Autodesk Inventor part; units mm, degrees
ref_plane "YZ Plane" through (0, 0, 0) normal (1, 0, 0) x (0, 1, 0)
ref_plane "XZ Plane" through (0, 0, 0) normal (0, 1, 0) x (-1, 0, 0)
ref_plane "XY Plane" through (0, 0, 0) normal (0, 0, 1) x (1, 0, 0)
sketch "Boceto1" plane through (0, 0, 0) normal (0, 0, 1) x (1, 0, 0)
  line L0 (0, 0) -> (130, 0)
  line L1 (130, 0) -> (130, -56.08)
  line L2 (130, -56.08) -> (0, -56.08)
  line L3 (0, -56.08) -> (0, 0)
  dimension "d0" = 130
  dimension "d1" = 56.08
extrude "Extrusión1" add sketch "Boceto1" along normal blind 5
sketch "Boceto2" plane through (0, 0, 5) normal (0, 0, 1) x (1, 0, 0)
  line L0 (130, 0) -> (130, -56.08)
  line L1 (0, -56.08) -> (0, 0)
  line L2 (130, -56.08) -> (0, -56.08)
  line L3 (16.75, -57.2435) -> (13.25, -57.2435)
  line L4 (13.25, -44.08) -> (16.75, -44.08)
  line L5 (116.75, -57.2435) -> (113.25, -57.2435)
  line L6 (113.25, -44.08) -> (116.75, -44.08)
  line L7 (12, -46.6661) -> (12, -49.2661)
  line L8 (18, -49.2661) -> (18, -46.6661)
  line L9 (112, -46.6661) -> (112, -49.2661)
  line L10 (118, -49.2661) -> (118, -46.6661)
  line L11 (12, -49.2661) -> (13.25, -49.2661)
  line L12 (16.75, -49.2661) -> (18, -49.2661)
  line L13 (16.75, -44.08) -> (16.75, -46.6661)
  line L14 (16.75, -49.2661) -> (16.75, -57.2435)
  line L15 (18, -46.6661) -> (16.75, -46.6661)
  line L16 (13.25, -46.6661) -> (12, -46.6661)
  line L17 (13.25, -57.2435) -> (13.25, -49.2661)
  line L18 (13.25, -46.6661) -> (13.25, -44.08)
  line L19 (112, -49.2661) -> (113.25, -49.2661)
  line L20 (116.75, -49.2661) -> (118, -49.2661)
  line L21 (116.75, -44.08) -> (116.75, -46.6661)
  line L22 (116.75, -49.2661) -> (116.75, -57.2435)
  line L23 (118, -46.6661) -> (116.75, -46.6661)
  line L24 (113.25, -46.6661) -> (112, -46.6661)
  line L25 (113.25, -57.2435) -> (113.25, -49.2661)
  line L26 (113.25, -46.6661) -> (113.25, -44.08)
  dimension "d7" = 6
  dimension "d8" = 12
  dimension "d14" = 13.25
  dimension "d15" = 1.25
  dimension "d16" = 1.25
  dimension "d17" = 13.25
  dimension "d18" = 3.5
extrude "Extrusión2" cut sketch "Boceto2" against normal blind 5
sketch "Boceto3" plane through (0, 0, 5) normal (0, 0, 1) x (1, 0, 0)
  line L0 (0, -56.08) -> (0, 0)
  line L1 (63.25, -6.5636) -> (63.25, 0.2503)
  line L2 (66.75, 0.2503) -> (66.75, -6.5636)
  line L3 (66.75, -6.5636) -> (68, -6.5636)
  line L4 (68, -6.5636) -> (68, -9.1636)
  line L5 (68, -9.1636) -> (66.75, -9.1636)
  line L6 (66.75, -9.1636) -> (66.75, -11.7497)
  line L7 (66.75, -11.7497) -> (63.25, -11.7497)
  line L8 (63.25, -11.7497) -> (63.25, -9.1636)
  line L9 (63.25, -9.1636) -> (62, -9.1636)
  line L10 (62, -9.1636) -> (62, -6.5636)
  line L11 (62, -6.5636) -> (63.25, -6.5636)
  line L12 (63.25, 0.2503) -> (66.75, 0.2503)
  dimension "d21" = 63.25
extrude "Extrusión3" cut sketch "Boceto3" against normal blind 5
fillet "Empalme1" radius 2 1 edges at (130, -56.08, 2.5)
fillet "Empalme2" radius 2 1 edges at (0, -56.08, 2.5)
sketch "Boceto4" plane through (0, 0, 5) normal (0, 0, 1) x (1, 0, 0)
  line L0 (113.25, -56.08) -> (16.75, -56.08)
  line L1 (0, -54.08) -> (0, 0)
  arc A0 (35, -18.08) -> (35, -38.08) centre (35, -28.08) ccw
  arc A1 (95, -38.08) -> (95, -18.08) centre (95, -28.08) ccw
  line L2 (35, -38.08) -> (95, -38.08)
  line L3 (95, -18.08) -> (35, -18.08)
  dimension "d26" = 20
  dimension "d27" = 20
  dimension "d28" = 60
  dimension "d29" = 35
  dimension "d30" = 28
extrude "Extrusión4" cut sketch "Boceto4" against normal blind 5
properties part number "pieza protectora 2"
For this review, take the finished solid that the model builds, in its own axes (mm). A direction names the side the tool comes from. Coordinates: 2 decimals unless noted, no trailing zeros. Write each loop counter-clockwise with the first axis right and the second up, starting at its lowest first coordinate (ties: lowest second). Pieces come first, ordered by that corner, then holes. Notation, with made-up numbers: (9, -8) -> (28, -8) arc R16 cw to (28, 18) -> close; hole circle Ø7 at (47, 34.5). An arc over 180 degrees is marked (long way). Write each question's results on one line, items separated by ' | '. Start each with the question number.
1) Consider section B-B (y = -28.08). Write out the cut boundary in (x, z), plus the area to 3 significant figures.
2) For faces 4 (the face through (18, -48, 3)), 5 (the face through (16.75, -53, 3)), 6 (the face through (63.25, -10, 3)), list the 3-axis set-ups (+Z, -Z, +X, -X, +Y, -Y) from which the entire face can be reached by the end or side of a thin tool; tool diameter is ignored.
3) Wall thickness on L1, parallel to X at y = -51, z = 2.8; L2, parallel to Y at x = 65, z = 3; L3, parallel to Y at x = 87.5, z = 1.4: over which ranges is each line inside the solid? List them lowest first. Write a range as [from, to].
4) Consider section A-A (x = 39). Write out the cut boundary in (y, z), plus the area to 3 significant figures.
5) The part is to be moulded in two halves that separate along Y. For faces 1 (the face through (65, -18.08, 3)), 2 (the face through (116.75, -53, 3)), 3 (the face through (15, -44.08, 3)), say which applies: +Y half, -Y half, draft (parallel to the pull), parting line (faces both ways), or undercut.
6) Insertion check: pin 1 (1.8 mm diameter, centred on x = 65.5, z = 3.5, fed in from +Y). The pin has a flat end and moves straight along its axis. Give the tip position at first contact, or say it passes through.
Geometry says:
1) outline: (0, 0) -> (25, 0) -> (25, 5) -> (0, 5) -> close; (105, 0) -> (130, 0) -> (130, 5) -> (105, 5) -> close | area: 250 mm^2
2) face 4: +Z, -Z | face 5: +Z, -Z, -Y | face 6: +Z, -Z, +Y
3) L1: [0, 13.25], [16.75, 113.25], [116.75, 130] | L2: [-56.08, -38.08], [-18.08, -11.75] | L3: [-56.08, -38.08], [-18.08, 0]
4) outline: (-56.08, 0) -> (-38.08, 0) -> (-38.08, 5) -> (-56.08, 5) -> close; (-18.08, 0) -> (0, 0) -> (0, 5) -> (-18.08, 5) -> close | area: 180 mm^2
5) face 1: undercut | face 2: draft | face 3: -Y half
6) pin 1: y = -11.75
